Here's the drawing with two shaded views (mm, measured from the low corner). I have some questions. Coordinates: 2 decimals unless noted, no trailing zeros. Write each loop counter-clockwise with the first axis right and the second up, starting at its lowest first coordinate (ties: lowest second). Pieces come first, ordered by that corner, then holes.
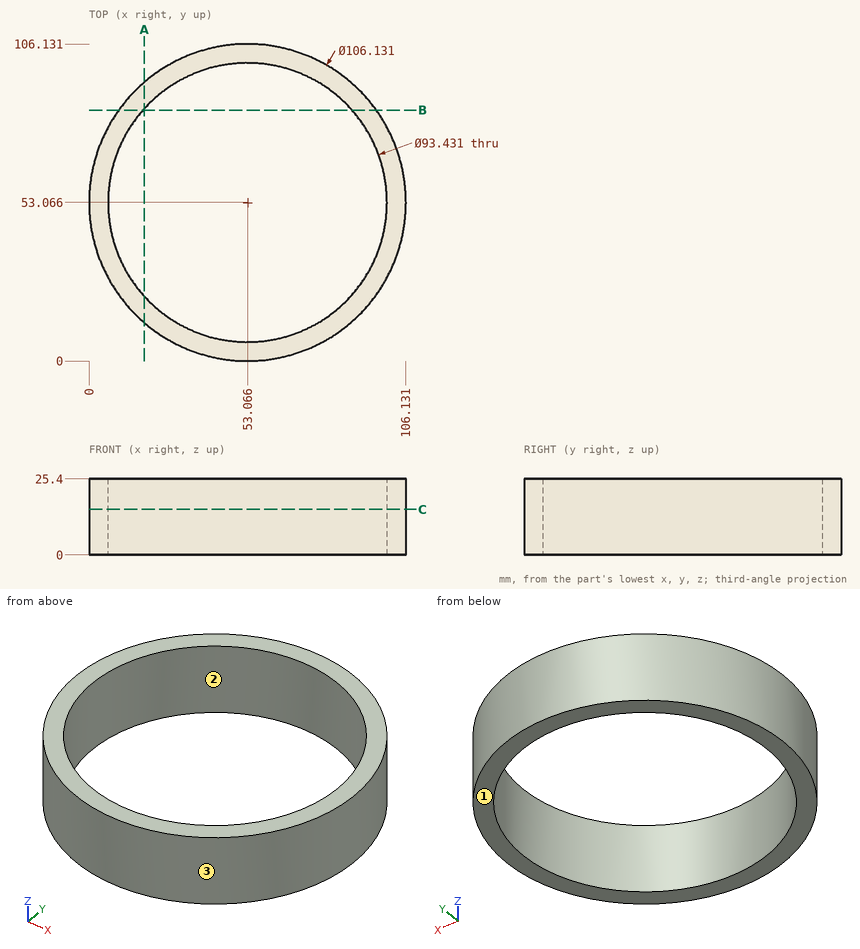
1. If we mould it in two halves opening along Y, with no side actions, what happens to the marked faces 1, 2 and 3? For each: pulls with the +Y half, pulls with the -Y half, needs draft (parallel to the pull), parting line crosses it, or undercut.
Verdict:
face 1: needs draft
face 2: undercut
face 3: parting line crosses it
2. I want a section at B-B on y = 84. Please give me the cut outline in (x, z).
Verdict:
outline: (9.95, 0) - (18.06, 0) - (18.06, 25.4) - (9.95, 25.4) - close; (88.07, 0) - (96.18, 0) - (96.18, 25.4) - (88.07, 25.4) - close
3. Please list where these lines run through material, in increasing order: line 1 along X through (y, z) = (53, 17); line 2 along Y through (x, z) = (82, 11.5); line 3 along X through (y, z) = (22.5, 24.25) (1 decimal).
Verdict:
line 1: x = 0 to 6.35, 99.78 to 106.13
line 2: y = 8.58 to 16.39, 89.74 to 97.55
line 3: x = 9.7 to 17.7, 88.4 to 96.4
4. I want a section at C-C on z = 15.25. Please give me the cut outline in (x, y) (1 decimal).
Verdict:
outline: circle Ø106.1 at (53.1, 53.1); hole circle Ø93.4 at (53.1, 53.1)
5. For pin 1 (5 mm diameter, centred on y = 88.5, z = 10, fed in from +X) (1 decimal); pin 2 (2 mm diameter, centred on y = 36, z = 14, fed in from -X); pin 3 (4 mm diameter, centred on x = 53, z = 6.5, fed in from +Y), each with a flat end and sliding along its axis, tell me the tip position at first contact or that it passes through.
Verdict:
pin 1: stops at x = 94.7
pin 2: stops at x = 2.49
pin 3: stops at y = 106.13
6. I want a section at A-A on x = 18.5. Please give me the cut outline in (y, z), plus the area to 3 significant figures.
Verdict:
outline: (12.8, 0) - (21.64, 0) - (21.64, 25.4) - (12.8, 25.4) - close; (84.49, 0) - (93.33, 0) - (93.33, 25.4) - (84.49, 25.4) - close
area: 449 mm2
